```python
from build123d import *

# Parameters (mm, degrees)
BOSS_EXTRUDE1_DEPTH = 3.175
SKETCH2_R           = 1.27
SKETCH2_R_2         = 1.4605
CUT_EXTRUDE1_DEPTH  = 149.140205971


with BuildPart() as part:
    # Sketch1 → Boss-Extrude1 (new body)
    with BuildSketch(Plane.XY):
        Polygon((0, 0), (0, 76.2), (127, 76.2), (127, 57.15), (19.05, 57.15), (19.05, 0), align=None)
    extrude(amount=BOSS_EXTRUDE1_DEPTH)

    # Sketch2 → Cut-Extrude1 (cut, through all)
    with BuildSketch(Plane.XY.offset(3.175)):
        with Locations((9.525, 9.525)):
            Circle(SKETCH2_R)
        with Locations((117.475, 66.675)):
            Circle(SKETCH2_R_2)
        with Locations((66.675, 66.675)):
            Circle(SKETCH2_R_2)
    extrude(amount=-CUT_EXTRUDE1_DEPTH, mode=Mode.SUBTRACT)


solid = part.part
```
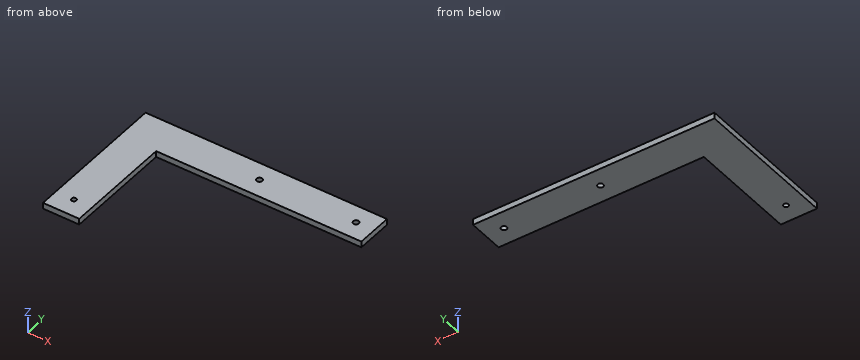
Model file for the job. Use its own axes, mm. Round coordinates to 2 decimals unless told otherwise and drop trailing zeros. Order: outer loops, then holes, each group sorted by start corner. A loop starts at its lowest first (then second) coordinate and runs counter-clockwise, first axis right, second up. Notation, with made-up numbers: (79, 36.25) -> (133, 36.25) arc R35 cw to (133, 69.25) -> close; hole circle Ø7 at (-7, 19.25). An arc over 180 degrees is marked (long way). Use one line per item in the form item = value.
Item 1: Cut at B-B, the plane y = 28. Write the cut outline in (x, z) (3 decimals), and give its area (3 significant figures).
Returned:
outline = (0, 0) -> (19.05, 0) -> (19.05, 3.175) -> (0, 3.175) -> close
area = 60.5 mm^2
Item 2: Drill centre lines: line 1 (X direction, y = 43, z = 1.7); line 2 (Y direction, x = 69, z = 0.8). Where is each one in solid material? Low to high.
Returned:
line_1 = 0 to 19.05
line_2 = 57.15 to 76.2
Item 3: Flat gauge pins, fed straight in: pin 1 Ø3 at (x, y) = (9.525, 9.525) entering from -Z; pin 2 Ø1 at (y, z) = (27.5, 2) entering from +X. Where does each tip first touch, or does it go through?
Returned:
pin_1 = 0
pin_2 = 19.05
Item 4: Cut at A-A, the plane z = 2.05. Give the number of separate pieces and of enclosed holes in the cut face, and give its area (3 significant figures).
Returned:
separate_pieces = 1
enclosed_holes = 3
area = 3,490 mm^2
Item 5: Cut at C-C, the plane x = 99. Write the cut outline in (y, z) (3 decimals).
Returned:
outline = (57.15, 0) -> (76.2, 0) -> (76.2, 3.175) -> (57.15, 3.175) -> close
